```python
from build123d import *

# Parameters (mm, degrees)
BOSS_EXTRUDE2_START  = -38.1
BOSS_EXTRUDE2_DEPTH  = 63.5
SKETCH2_W            = 41.6814
SKETCH2_H            = 3.175
BOSS_EXTRUDE3_DEPTH  = 38.1
SKETCH3_W            = 5.08
SKETCH3_H            = 25.4
BOSS_EXTRUDE4_DEPTH  = 76.2
SKETCH4_W            = 3.175
SKETCH4_H            = 7.398582519
BOSS_EXTRUDE5_DEPTH  = 38.1
SKETCH5_W            = 25.4
SKETCH5_H            = 5.075789281
BOSS_EXTRUDE6_DEPTH  = 95.25
FILLET1_R            = 2.54
CUT_EXTRUDE1_DEPTH   = 5.075789281
CUT_EXTRUDE2_DEPTH   = 5.08
FILLET1_OF_MIRROR5_R = 2.54
FILLET3_R            = 2.54
SKETCH9_R            = 9.525
CUT_EXTRUDE3_DEPTH   = 50.8
SKETCH11_R           = 6.35
CUT_EXTRUDE4_DEPTH   = 166.904133083
SKETCH12_R           = 6.35
CUT_EXTRUDE5_DEPTH   = 175.78091679


with BuildPart() as part:
    # Sketch1 → Boss-Extrude2 (new body)
    with BuildSketch(Plane(origin=(0, 0, 0), x_dir=(1, 0, 0), z_dir=(0, 1, 0)).offset(BOSS_EXTRUDE2_START)):
        Polygon((46.7614, 3.175), (46.7614, 0), (66.0370282, 0), (66.0370282, 19.2756282), (62.8620282, 19.2756282), align=None)
    boss_extrude2 = extrude(amount=BOSS_EXTRUDE2_DEPTH)

    # Sketch2 → Boss-Extrude3 (add)
    with BuildSketch(Plane(origin=(0, 0, 0), x_dir=(1, 0, 0), z_dir=(0, 1, 0))):
        with Locations((25.9207, 1.5875)):
            Rectangle(SKETCH2_W, SKETCH2_H)
    boss_extrude3 = extrude(amount=-BOSS_EXTRUDE3_DEPTH)

    # Sketch3 → Boss-Extrude4 (add)
    with BuildSketch(Plane(origin=(0, 0, 0), x_dir=(1, 0, 0), z_dir=(0, 1, 0))):
        with Locations((2.54, 12.7)):
            Rectangle(SKETCH3_W, SKETCH3_H)
    boss_extrude4 = extrude(amount=-BOSS_EXTRUDE4_DEPTH)

    # Sketch4 → Boss-Extrude5 (add)
    with BuildSketch(Plane(origin=(0, 0, 0), x_dir=(1, 0, 0), z_dir=(0, 1, 0))):
        with Locations((64.4495282, 22.97491946)):
            Rectangle(SKETCH4_W, SKETCH4_H)
    boss_extrude5 = extrude(amount=-BOSS_EXTRUDE5_DEPTH)

    # Sketch5 → Boss-Extrude6 (add)
    with BuildSketch(Plane(origin=(0, 0, 0), x_dir=(1, 0, 0), z_dir=(0, 1, 0))):
        with Locations((53.3370282, 29.21210536)):
            Rectangle(SKETCH5_W, SKETCH5_H)
    boss_extrude6 = extrude(amount=-BOSS_EXTRUDE6_DEPTH)

    # Fillet1
    fillet1_edges = [part.edges().sort_by_distance(p)[0] for p in [
        (5.08, -19.05, -3.175),
        (46.7614, 0, -1.5875),
        (62.8620282, -19.05, -26.674210719),
    ]]
    fillet(fillet1_edges, radius=FILLET1_R)

    # Sketch7 → Cut-Extrude1 (cut)
    with BuildSketch(Plane(origin=(0, 0, -31.75), x_dir=(-1, 0, 0), z_dir=(0, 0, -1))):
        Polygon((-40.6370282, -82.55), (-53.3370282, -95.25), (-40.6370282, -95.25), align=None)
    cut_extrude1 = extrude(amount=-CUT_EXTRUDE1_DEPTH, mode=Mode.SUBTRACT)

    # Sketch8 → Cut-Extrude2 (cut)
    with BuildSketch(Plane.ZY):
        Polygon((-25.4, -76.2), (-25.4, -63.5), (-12.7, -76.2), align=None)
    cut_extrude2 = extrude(amount=-CUT_EXTRUDE2_DEPTH, mode=Mode.SUBTRACT)

    # Mirror5: Boss-Extrude2, Boss-Extrude3, Boss-Extrude4, Boss-Extrude5, Boss-Extrude6, Cut-Extrude1, Cut-Extrude2 across plane
    add(boss_extrude2.mirror(Plane(origin=(0, -38.1, 0), x_dir=(1, 0, 0), z_dir=(0, 0, 1))))
    add(boss_extrude3.mirror(Plane(origin=(0, -38.1, 0), x_dir=(1, 0, 0), z_dir=(0, 0, 1))))
    add(boss_extrude4.mirror(Plane(origin=(0, -38.1, 0), x_dir=(1, 0, 0), z_dir=(0, 0, 1))))
    add(boss_extrude5.mirror(Plane(origin=(0, -38.1, 0), x_dir=(1, 0, 0), z_dir=(0, 0, 1))))
    add(boss_extrude6.mirror(Plane(origin=(0, -38.1, 0), x_dir=(1, 0, 0), z_dir=(0, 0, 1))))
    add(cut_extrude1.mirror(Plane(origin=(0, -38.1, 0), x_dir=(1, 0, 0), z_dir=(0, 0, 1))), mode=Mode.SUBTRACT)
    add(cut_extrude2.mirror(Plane(origin=(0, -38.1, 0), x_dir=(1, 0, 0), z_dir=(0, 0, 1))), mode=Mode.SUBTRACT)

    # Fillet1 of Mirror5
    fillet1_of_mirror5_edges = [part.edges().sort_by_distance(p)[0] for p in [
        (5.08, -19.05, 3.175),
        (46.7614, 0, 1.5875),
        (62.8620282, -19.05, 26.674210719),
    ]]
    fillet(fillet1_of_mirror5_edges, radius=FILLET1_OF_MIRROR5_R)

    # Mirror6: part across plane


with BuildPart() as part_1:
    add(part.part)
    add(part.part.mirror(Plane(origin=(66.0370282, -38.1, 0), x_dir=(0, 0, 1), z_dir=(1, 0, 0))))

    # Fillet3
    fillet3_edges = [part_1.edges().sort_by_distance(p)[0] for p in [
        (66.0370282, 0, 19.2756282),
        (66.0370282, 0, -19.2756282),
    ]]
    fillet(fillet3_edges, radius=FILLET3_R)

    # Sketch9 → Cut-Extrude3 (cut)
    with BuildSketch(Plane(origin=(0, 25.4, 0), x_dir=(1, 0, 0), z_dir=(0, 1, 0))):
        with Locations(Location((66.0370282, 0, 0), (0, 0, 270))):
            Circle(SKETCH9_R)
    extrude(amount=-CUT_EXTRUDE3_DEPTH, mode=Mode.SUBTRACT)

    # Sketch11 → Cut-Extrude4 (cut, through all)
    with BuildSketch(Plane(origin=(132.0740564, 0, 0), x_dir=(0, 0, -1), z_dir=(1, 0, 0))):
        with Locations((0, -50.8)):
            Circle(SKETCH11_R)
    extrude(amount=-CUT_EXTRUDE4_DEPTH, mode=Mode.SUBTRACT)

    # Sketch12 → Cut-Extrude5 (cut, through all)
    with BuildSketch(Plane.XY.offset(31.75)):
        with Locations((66.0370282, -69.85)):
            Circle(SKETCH12_R)
    extrude(amount=-CUT_EXTRUDE5_DEPTH, mode=Mode.SUBTRACT)


solid = part_1.part
```
Here's how the part is built. I have some questions about the finished solid (model axes, mm). A direction names the side the tool comes from. Give positions to 0.01 mm unless a question says otherwise; leave off trailing zeros. Write each loop counter-clockwise with the first axis right and the second up, starting at its lowest first coordinate (ties: lowest second). Pieces come first, ordered by that corner, then holes. Notation, with made-up numbers: (12.5, 55) -> (69.5, 55) arc R8 cw to (69.5, 67) -> close; hole circle Ø5 at (85, 82). An arc over 180 degrees is marked (long way). Use one line per item in the form item = value.
1) On a 3-axis mill with a long thin cutter (end or side, diameter ignored), from which of +Z, -Z, +X, -X, +Y, -Y can I reach the whole of each face in a straight line? I mean faces 4 (the face through (130, -31, 25.4)), 5 (the face through (40.637, -41, -29)), 6 (the face through (130, -31, -25.4)). Say none if no direction works.
Verdict:
face_4 = +Z, +X, +Y, -Y
face_5 = -Z, -X, +Y, -Y
face_6 = -Z, +X, +Y, -Y
2) If I drill on L1, parallel to Y at x = 128, z = 0; L2, parallel to X at y = -20, z = 17; L3, parallel to Z at x = 58, y = -31.5, over which ranges is the centre line in solid material (lowest first)? Write a range as [from, to].
Verdict:
L1 = [-76.2, -57.15], [-44.45, 0]
L2 = [0, 5.08], [60.59, 71.49], [126.99, 132.07]
L3 = [-31.75, -26.67], [-14.41, 14.41], [26.67, 31.75]
3) Suppose I cut it at D-D (x = 94.5). Please give me the cut outline in (y, z) (3 decimals), and give its area (3 significant figures).
Verdict:
outline = (-38.1, -3.175) -> (0, -3.175) -> (0, 3.175) -> (-38.1, 3.175) -> close
area = 242 mm2
4) I'm going to push flat-ended pins straight in: pin 1 (5.5 mm diameter, centred on x = 128.5, y = -43.5, fed in from +Z); pin 2 (1.5 mm diameter, centred on x = 129, y = -38, fed in from -Z); pin 3 (5.5 mm diameter, centred on y = -20.5, z = 30.5, fed in from -X). Where does each tip first touch, or does it pass through?
Verdict:
pin_1 = 25.4
pin_2 = -25.4
pin_3 = 40.64
5) Suppose I cut it at B-B (x = 50.5). Please give me the cut outline in (y, z).
Verdict:
outline = (-92.41, -31.75) -> (0, -31.75) -> (0, -26.67) -> (-92.41, -26.67) -> close; (-92.41, 26.67) -> (0, 26.67) -> (0, 31.75) -> (-92.41, 31.75) -> close; (-38.1, -6.91) -> (25.4, -6.91) -> (25.4, 6.91) -> (-38.1, 6.91) -> close
6) Suppose I cut it at C-C (y = 13). Please give me the cut outline in (x, z) (3 decimals), and give its area (3 significant figures).
Verdict:
outline = (46.761, -3.175) -> (62.862, -19.276) -> (69.212, -19.276) -> (85.313, -3.175) -> (85.313, 3.175) -> (69.212, 19.276) -> (62.862, 19.276) -> (46.761, 3.175) -> close; hole circle Ø19.05 at (66.037, 0)
area = 683 mm2
7) Suppose I cut it at A-A (y = -60). Please give me the cut outline in (x, z), and give its area (3 significant figures).
Verdict:
outline = (0, -25.4) -> (5.08, -25.4) -> (5.08, 25.4) -> (0, 25.4) -> close; (40.64, -31.75) -> (91.44, -31.75) -> (91.44, -26.67) -> (40.64, -26.67) -> close; (40.64, 26.67) -> (91.44, 26.67) -> (91.44, 31.75) -> (40.64, 31.75) -> close; (126.99, -25.4) -> (132.07, -25.4) -> (132.07, 25.4) -> (126.99, 25.4) -> close
area = 1,030 mm2
8) We'd pull the mould along Y, two halves only. Please class faces 1 (the face through (105, -17, 3.175)), 2 (the face through (2.6, -44.5, 0.8)), 3 (the face through (66, -95.25, -29)): +Y half, -Y half, draft (parallel to the pull), parting line (faces both ways), or undercut.
Verdict:
face_1 = draft
face_2 = undercut
face_3 = -Y half
